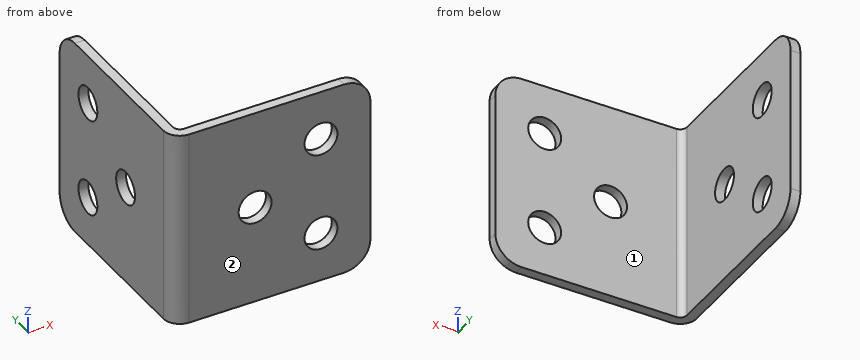
from build123d import *

# Parameters (mm, degrees)
EXTRUDE_1_DEPTH     = 30
SKETCH_2_R          = 2.5
CUT_EXTRUDE_1_DEPTH = 40
SKETCH_3_R          = 2.5
CUT_EXTRUDE_2_DEPTH = 40
FILLET_1_R          = 4


with BuildPart() as part:
    # Эскиз1 → Бобышка-Вытянуть1 (new body)
    with BuildSketch(Plane.XY):
        with BuildLine():
            Line((-2.5, 27.5), (-2.5, 0))
            ThreePointArc((-2.5, 0), (-1.767766953, -1.767766953), (0, -2.5))
            Line((0, -2.5), (27.5, -2.5))
            Line((27.5, -2.5), (27.5, -1))
            Line((27.5, -1), (0, -1))
            ThreePointArc((0, -1), (-0.707106781, -0.707106781), (-1, 0))
            Line((-1, 0), (-1, 27.5))
            Line((-1, 27.5), (-2.5, 27.5))
        make_face()
    extrude(amount=EXTRUDE_1_DEPTH)

    # Эскиз2 → Вырез-Вытянуть1 (cut)
    with BuildSketch(Plane.ZY.offset(2.5)):
        with Locations(Location((7.5, 20, 0), (0, 0, 270))):
            Circle(SKETCH_2_R)
        with Locations(Location((22.5, 20, 0), (0, 0, 270))):
            Circle(SKETCH_2_R)
        with Locations(Location((15, 10, 0), (0, 0, 270))):
            Circle(SKETCH_2_R)
    extrude(amount=-CUT_EXTRUDE_1_DEPTH, mode=Mode.SUBTRACT)

    # Эскиз3 → Вырез-Вытянуть2 (cut)
    with BuildSketch(Plane.XZ.offset(2.5)):
        with Locations((20, 7.5)):
            Circle(SKETCH_3_R)
        with Locations((20, 22.5)):
            Circle(SKETCH_3_R)
        with Locations((10, 15)):
            Circle(SKETCH_3_R)
    extrude(amount=-CUT_EXTRUDE_2_DEPTH, mode=Mode.SUBTRACT)

    # Скругление1
    fillet_1_edges = [part.edges().sort_by_distance(p)[0] for p in [
        (-1.75, 27.5, 0),
        (27.5, -1.75, 30),
        (-1.75, 27.5, 30),
        (27.5, -1.75, 0),
    ]]
    fillet(fillet_1_edges, radius=FILLET_1_R)


solid = part.part
The listing builds one solid part. Answer for the finished solid, in the listing's coordinates (mm). Face numbers are marked on the shaded views. A direction names the side the tool comes from. Give positions to 0.01 mm unless a question says otherwise; leave off trailing zeros. Write each loop counter-clockwise with the first axis right and the second up, starting at its lowest first coordinate (ties: lowest second). Pieces come first, ordered by that corner, then holes.
1) Section D-D (y = 20) is taken. Write down the section's boundary in (x, z).
2) Find the intervals of material crossed by L1, parallel to Z at x = 20, y = -2.1; L2, parallel to X at y = 18, z = 2.25, in increasing order.
3) Section B-B (z = 13) is taken. Write down the section's boundary in (x, y), and give its area (3 significant figures).
4) A tool of negligible diameter and unlimited length cuts with its end or side. For the marked faces 1 and 2, from which of +Z, -Z, +X, -X, +Y, -Y can it reach the whole face along a straight path? Write none if from no direction.
5) Section A-A (y = 10) is taken. Write down the section's boundary in (x, z), and give its area (3 significant figures).
6) Given P1, Ø1.5, axis at x = 10.5, z = 5, coming from the +Y side; P2, Ø14, axis at y = 19, z = 10.5, coming from the +X side, each flat-ended and moving along its own axis, determine where each tip first touches the part or whether it passes through.
Response:
1. outline: (-2.5, 0) - (-1, 0) - (-1, 5) - (-2.5, 5) - close; (-2.5, 10) - (-1, 10) - (-1, 20) - (-2.5, 20) - close; (-2.5, 25) - (-1, 25) - (-1, 30) - (-2.5, 30) - close
2. L1: z = 0 to 5, 10 to 20, 25 to 30
2. L2: x = -2.5 to -1
3. outline: (-2.5, 0) arc R2.5 ccw to (0, -2.5) - (8.5, -2.5) - (8.5, -1) - (0, -1) arc R1 cw to (-1, 0) - (-1, 8.5) - (-2.5, 8.5) - close; (-2.5, 11.5) - (-1, 11.5) - (-1, 27.5) - (-2.5, 27.5) - close; (11.5, -2.5) - (27.5, -2.5) - (27.5, -1) - (11.5, -1) - close
3. area: 77.6 mm2
4. face 1: +Z, -Z, +X, +Y
4. face 2: +Z, -Z, +X, -X, -Y
5. outline: (-2.5, 0) - (-1, 0) - (-1, 12.5) - (-2.5, 12.5) - close; (-2.5, 17.5) - (-1, 17.5) - (-1, 30) - (-2.5, 30) - close
5. area: 37.5 mm2
6. P1: stops at y = -1
6. P2: stops at x = -1
